Job drawing, mm, ordinate dimensions from the low corner. One solid piece. A direction names the side the tool comes from. Round coordinates to 2 decimals unless told otherwise and drop trailing zeros. Loops run counter-clockwise (first coordinate to the right, second up) from the corner with the lowest first, then second, coordinate; pieces in that order, holes last. Notation, with made-up numbers: M 36.5,63.5 L 61.5,63.5 A22 cw 61.5,85.5 Z; hole C 84.5,83 d5. An arc over 180 degrees is marked long. Use a Markdown table: item, result. Add a question column.
(1) Two-plate mould, pull along X, no slides. Class the marked faces 1, 2, 3 and 4: released by +X, released by -X, zero draft, split by the parting line, or undercut.
(2) Band-saw the part on B-B, the plane z = 2.25. Write the cut outline in (x, y).
(3) Band-saw the part on D-D, the plane x = 39.5. Write the cut outline in (y, z), and give its area (3 significant figures).
(4) Band-saw the part on A-A, the plane x = 22.5. Write the cut outline in (y, z).
(5) Wall check: L1, parallel to Y at x = 22.5, z = 3.5; L2, parallel to X at y = 18, z = 4; L3, parallel to Y at x = 8, z = 14. Give the ranges that are in metal, low to high.
(6) Which spindle directions (+Z, -Z, +X, -X, +Y, -Y) get a long thin tool onto all of the face, cutting with end or side? Do the marked faces 5 and 6. Say none if no direction does.
(7) Band-saw the part on C-C, the plane y = 23. Write the cut outline in (x, z), and give its area (3 significant figures).
(8) Flat gauge pins, fed straight in: P1, Ø13, axis at x = 22.5, y = 18, coming from the +Z side; P2, Ø2, axis at x = 7, z = 11, coming from the -Y side; P3, Ø6, axis at x = 31, z = 8, coming from the +Y side; P4, Ø4.5, axis at x = 33, y = 1, coming from the +Z side. Where does each tip first touch, or does it go through?
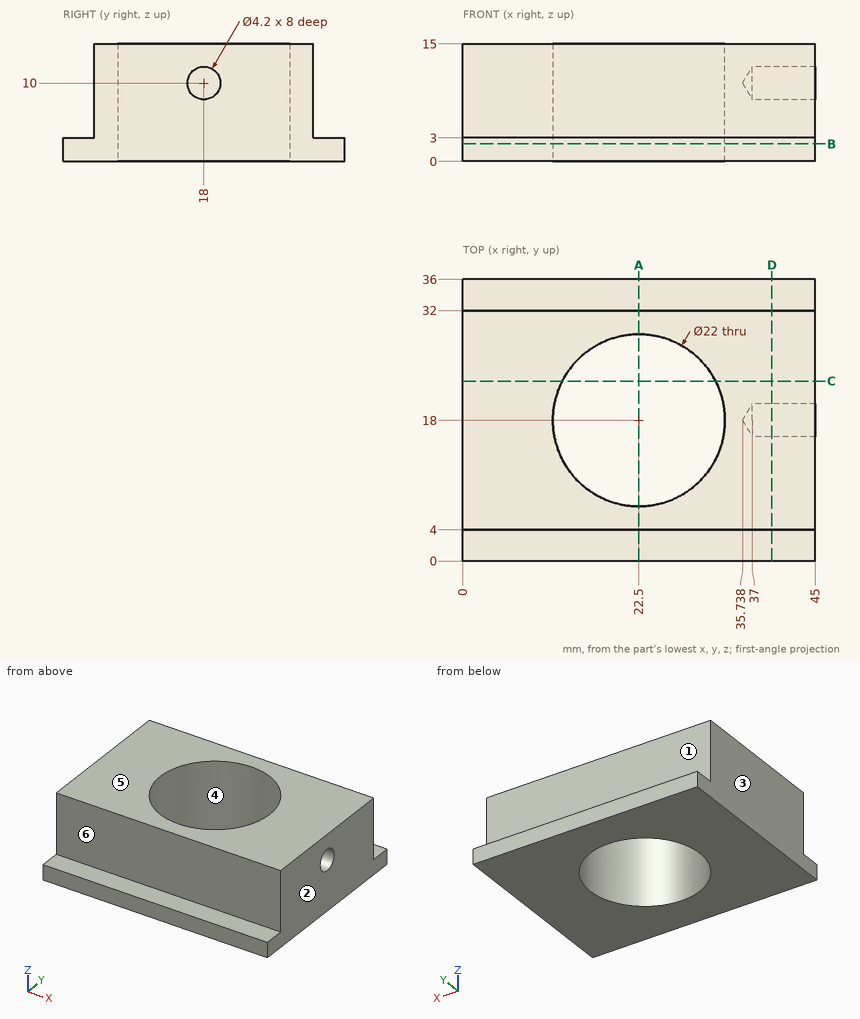
Return value:
| question | item | result |
|---|---|---|
| 1 | face 1 | zero draft |
| 1 | face 2 | released by +X |
| 1 | face 3 | released by -X |
| 1 | face 4 | undercut |
| 2 | outline | M 0,0 L 45,0 L 45,36 L 0,36 Z; hole C 22.5,18 d22 |
| 3 | outline | M 0,0 L 36,0 L 36,3 L 32,3 L 32,15 L 4,15 L 4,3 L 0,3 Z; hole C 18,10 d4.2 |
| 3 | area | 430 mm^2 |
| 4 | outline | M 0,0 L 7,0 L 7,15 L 4,15 L 4,3 L 0,3 Z; M 29,0 L 36,0 L 36,3 L 32,3 L 32,15 L 29,15 Z |
| 5 | L1 | 4 to 7, 29 to 32 |
| 5 | L2 | 0 to 11.5, 33.5 to 45 |
| 5 | L3 | 4 to 32 |
| 6 | face 5 | +Z, +X, -X, +Y, -Y |
| 6 | face 6 | +Z, +X, -X, -Y |
| 7 | outline | M 0,0 L 12.7,0 L 12.7,15 L 0,15 Z; M 32.3,0 L 45,0 L 45,15 L 32.3,15 Z |
| 7 | area | 381 mm^2 |
| 8 | P1 | through |
| 8 | P2 | y = 4 |
| 8 | P3 | y = 32 |
| 8 | P4 | z = 3 |
